from build123d import *


with BuildPart() as part:
    # Sketch1 → Revolve1 (revolve)
    with BuildSketch(Plane.XY, mode=Mode.PRIVATE) as revolve1_sk:
        with BuildLine():
            Line((-5.8, 9), (-5.8, 8.75))
            Line((-5.8, 8.75), (-5.6, 8.75))
            Line((-5.6, 8.75), (-5.6, 9))
            Line((-5.6, 9), (-5.6, 12.851513548))
            Line((-5.6, 12.851513548), (-5, 14.5))
            Line((-5, 14.5), (-5, 15.1))
            ThreePointArc((-5, 15.1), (-5.4, 15.5), (-5.8, 15.1))
            Line((-5.8, 15.1), (-5.8, 14.5))
            Line((-5.8, 14.5), (-5.6, 14.5))
            Line((-5.6, 14.5), (-5.6, 15.1))
            ThreePointArc((-5.6, 15.1), (-5.4, 15.3), (-5.2, 15.1))
            Line((-5.2, 15.1), (-5.2, 14.535265396))
            Line((-5.2, 14.535265396), (-5.8, 12.886778944))
            Line((-5.8, 12.886778944), (-5.8, 9))
        make_face()
    revolve(revolve1_sk.sketch.rotate(Axis((-6, 0, 0), (1, 0, 0)), 90), axis=Axis((-6, 0, 0), (1, 0, 0)))


solid = part.part
For this review, take the finished solid that the model builds, in its own axes (mm). A direction names the side the tool comes from. Give positions to 0.01 mm unless a question says otherwise; leave off trailing zeros. Loops run counter-clockwise (first coordinate to the right, second up) from the corner with the lowest first, then second, coordinate; pieces in that order, holes last. Notation, with made-up numbers: M 75,54 L 119,54 A17 cw 119,74 Z; hole C 67,89 d8. An arc over 180 degrees is marked long. Answer as a JSON object with one key per item and string values. Group by question number.
Q1. Add section C-C on x = -5.45. Give the boundary of the cut face in (y, z), and give its area (3 significant figures).
Q2. Tool access review of faces 1 (the flat face through (-5.6, -3, -8.4)), 2 (the flat face through (-5.8, 8.4, -3)): name each direction out of +Z, -Z, +X, -X, +Y, -Y from which nothing blocks a thin tool from reaching the whole face with its end or side.
Q3. For probe 1 along X at (y, z) = (3.5, -9.5); probe 2 along X at (y, z) = (13.5, -7); probe 3 along X at (y, z) = (2, -13.5), list the stretches that pass through material, from the lowest coordinate up. Write a range as [from, to].
Q4. Add section A-A on z = 0. Give the boundary of the cut face in (x, y).
Q5. Insertion check: P1, Ø10, axis at y = 2.5, z = -2.5, coming from the +X side. The pin has a flat end and moves straight along its axis. Give the tip position at first contact, or say it passes through.
Q6. Mouldability with a two-part tool opening along X and no side actions: class faces 3 (the flat face through (-5.2, -12.4, -7.9)), 4 (the flat face through (-5.8, -13.5, -5.7)), 5 (the flat face through (-5.6, -5.7, 13.5)), 6 (the flat face through (-5, -5.7, 13.5)) as +X half, -X half, draft (parallel to the pull), parting line (faces both ways), or undercut.
Checked values:
{
 "1": {"outline": "C 0,0 d30.99; C 0,0 d27.7; hole C 0,0 d30.59; hole C 0,0 d26.53", "area": "69.5 mm²"},
 "2": {"face 1": "+X", "face 2": "+Z, -Z, -X, +Y, -Y"},
 "3": {"probe 1": "[-5.8, -5.6]", "probe 2": "[-5.79, -5.57], [-5.23, -5.01]", "probe 3": "[-5.52, -5.31]"},
 "4": {"outline": "M -5.8,-15.1 A0.4 ccw -5,-15.1 L -5,-14.5 L -5.6,-12.85 L -5.6,-8.75 L -5.8,-8.75 L -5.8,-12.89 L -5.2,-14.54 L -5.2,-15.1 A0.2 cw -5.6,-15.1 L -5.6,-14.5 L -5.8,-14.5 Z; M -5.8,8.75 L -5.6,8.75 L -5.6,12.85 L -5,14.5 L -5,15.1 A0.4 ccw -5.8,15.1 L -5.8,14.5 L -5.6,14.5 L -5.6,15.1 A0.2 cw -5.2,15.1 L -5.2,14.54 L -5.8,12.89 Z"},
 "5": {"P1": "through"},
 "6": {"face 3": "undercut", "face 4": "-X half", "face 5": "undercut", "face 6": "+X half"}
}
